CAD build for the part. Positions are in the model's coordinates, mm. A direction names the side the tool comes from. Give positions to 0.01 mm unless a question says otherwise; leave off trailing zeros. Loops run counter-clockwise (first coordinate to the right, second up) from the corner with the lowest first, then second, coordinate; pieces in that order, holes last.
Item 1: Saw through at C-C on z = -5.5. Give the number of separate pieces and of enclosed holes in the cut face, plus the area to 3 significant figures.
Item 2: Probe probe 1 along X at (y, z) = (24.5, -7); probe 2 along X at (y, z) = (35.5, -4.25); probe 3 along Y at (x, z) = (19.5, -4) (3 decimals). List the from-to ranges inside material, lowest first.
Item 3: Drop flat-ended pins along their axis: P1, Ø2, axis at y = 38, z = -2, coming from the -X side; P2, Ø2.5, axis at x = 9.35, y = 18.04, coming from the +Z side; P3, Ø1.6, axis at x = -9.35, y = 18.04, coming from the -Z side. Give the stop position or say it passes through.
Item 4: Which spindle directions (+Z, -Z, +X, -X, +Y, -Y) get a long thin tool onto all of the face, cutting with end or side? Do faces 1 (the flat face through (-25.4, 3, -5)), 2 (the cylindrical face through (-13.424, 50.221, -6.502)), 3 (the cylindrical face through (24.37, 52.895, -7.021)), 4 (the cylindrical face through (4.44, 8.16, -4.7)). Say none if no direction does.
Item 5: Mould opens along Y. For faces 5 (the cylindrical face through (24.05, 3.22, -5.2)), 6 (the cylindrical face through (18.22, 57.83, -4.7)), 7 (the flat face through (0, 67, -7)) say: released by +Y, released by -Y, zero draft, split by the parting line, or undercut.
Item 6: Saw through at B-B on y = 36. Give the cut face in (x, z) (3 decimals), plus the area to 3 significant figures.
Item 7: Saw through at A-A on y = 59.38. Give the cut face in (x, z) (3 decimals), plus the area to 3 significant figures.
from build123d import *

# Parameters (mm, degrees)
SKETCH1_R                 = 1.5875
EXTRUDE1_DEPTH            = 9.525
SKETCH2_W                 = 12.7
SKETCH2_H                 = 44.635078528
CUT_EXTRUDE1_DEPTH        = 73.561511865
FILLET1_R                 = 6.35
CHAMFER1_SIZE             = 4.445
FILLET2_R                 = 6.35
FILLET3_R                 = 6.35
SKETCH3_R                 = 2.000000064
CUT_EXTRUDE2_DEPTH        = 67.742756192
SKETCH4_R                 = 1.016
EXTRUDE2_DEPTH            = 73.561511865
LPATTERN1_COUNT           = 3
LPATTERN1_PITCH           = 6.35
LPATTERN1_COPY_1_SKETCH_R = 1.016
LPATTERN1_COPY_1_DEPTH    = 73.561511865
LPATTERN1_COPY_2_SKETCH_R = 1.016
LPATTERN1_COPY_2_DEPTH    = 73.561511865
FILLET5_R                 = 2.54


with BuildPart() as part:
    # Sketch1 → Extrude1 (new body)
    with BuildSketch(Plane.XY):
        with BuildLine():
            Line((26.18105, 50.985078528), (26.18105, 61.92))
            ThreePointArc((26.18105, 61.92), (24.693152448, 65.512102448), (21.10105, 67))
            Line((21.10105, 67), (-21.10105, 67))
            ThreePointArc((-21.10105, 67), (-24.693152448, 65.512102448), (-26.18105, 61.92))
            Line((-26.18105, 61.92), (-26.18105, 50.985078528))
            Line((-26.18105, 50.985078528), (-12.7, 50.985078528))
            Line((-12.7, 50.985078528), (-12.7, 6.35))
            Line((-12.7, 6.35), (-25.4, 6.35))
            Line((-25.4, 6.35), (-25.4, 0))
            Line((-25.4, 0), (25.4, 0))
            Line((25.4, 0), (25.4, 6.35))
            Line((25.4, 6.35), (12.7, 6.35))
            Line((12.7, 6.35), (12.7, 50.985078528))
            Line((12.7, 50.985078528), (26.18105, 50.985078528))
        make_face()
        with Locations((-18.56105, 59.38)):
            Circle(SKETCH1_R, mode=Mode.SUBTRACT)
        with Locations((18.56105, 59.38)):
            Circle(SKETCH1_R, mode=Mode.SUBTRACT)
    extrude(amount=-EXTRUDE1_DEPTH)

    # Sketch2 → Cut-Extrude1 (cut, through all)
    with BuildSketch(Plane(origin=(0, 0, -9.525), x_dir=(-1, 0, 0), z_dir=(0, 0, -1))):
        with Locations((0, 28.667539264)):
            Rectangle(SKETCH2_W, SKETCH2_H)
    extrude(amount=-CUT_EXTRUDE1_DEPTH, mode=Mode.SUBTRACT)

    # Fillet1
    fillet1_edges = [part.edges().sort_by_distance(p)[0] for p in [
        (-26.18105, 50.985078528, -4.7625),
        (26.18105, 50.985078528, -4.7625),
    ]]
    fillet(fillet1_edges, radius=FILLET1_R)

    # Chamfer1
    chamfer1_edges = [part.edges().sort_by_distance(p)[0] for p in [
        (-16.265525, 50.985078528, 0),
        (-26.18105, 59.627539264, 0),
        (16.265525, 50.985078528, 0),
        (0, 67, 0),
        (26.18105, 59.627539264, 0),
    ]]
    chamfer(chamfer1_edges, length=CHAMFER1_SIZE)

    # Fillet2
    fillet2_edges = [part.edges().sort_by_distance(p)[0] for p in [
        (6.35, 50.985078528, -4.7625),
        (-6.35, 50.985078528, -4.7625),
        (6.35, 6.35, -4.7625),
        (-6.35, 6.35, -4.7625),
    ]]
    fillet(fillet2_edges, radius=FILLET2_R - 0.0001)  # a hair under: the kernel refuses the full size

    # Fillet3
    fillet3_edges = [part.edges().sort_by_distance(p)[0] for p in [
        (-12.7, 6.35, -4.7625),
        (12.7, 6.35, -4.7625),
    ]]
    fillet(fillet3_edges, radius=FILLET3_R)

    # Sketch3 → Cut-Extrude2 (cut, through all)
    with BuildSketch(Plane(origin=(0, 6.35, 0), x_dir=(1, 0, 0), z_dir=(0, 1, 0))):
        with Locations(Location((-22.098, 4.7625, 0), (0, 0, 270))):
            Circle(SKETCH3_R)
    cut_extrude2 = extrude(amount=-CUT_EXTRUDE2_DEPTH, mode=Mode.SUBTRACT)

    # Mirror2: Cut-Extrude2 across plane
    add(cut_extrude2.mirror(Plane(origin=(0, 0, 0), x_dir=(0, 0, 1), z_dir=(1, 0, 0))), mode=Mode.SUBTRACT)

    # Sketch4 → Extrude2 (cut, through all)
    with BuildSketch(Plane.XY):
        with Locations((9.345089473, 30.742631811)):
            Circle(SKETCH4_R)
    extrude2 = extrude(amount=-EXTRUDE2_DEPTH, mode=Mode.SUBTRACT)

    # Mirror3: Extrude2 across plane
    add(extrude2.mirror(Plane(origin=(0, 0, 0), x_dir=(0, 0, 1), z_dir=(1, 0, 0))), mode=Mode.SUBTRACT)

    # LPattern1: Extrude2 ×3
    with Locations(*[(0, -i * LPATTERN1_PITCH, 0) for i in range(1, LPATTERN1_COUNT)]):
        add(extrude2, mode=Mode.SUBTRACT)

    # LPattern1 copy 1 sketch → LPattern1 copy 1 (cut, through all)
    with BuildSketch(Plane(origin=(0, -6.35, 0), x_dir=(-1, 0, 0), z_dir=(0, 0, 1))):
        with Locations((9.345089473, -30.742631811)):
            Circle(LPATTERN1_COPY_1_SKETCH_R)
    extrude(amount=-LPATTERN1_COPY_1_DEPTH, mode=Mode.SUBTRACT)

    # LPattern1 copy 2 sketch → LPattern1 copy 2 (cut, through all)
    with BuildSketch(Plane(origin=(0, -12.7, 0), x_dir=(-1, 0, 0), z_dir=(0, 0, 1))):
        with Locations((9.345089473, -30.742631811)):
            Circle(LPATTERN1_COPY_2_SKETCH_R)
    extrude(amount=-LPATTERN1_COPY_2_DEPTH, mode=Mode.SUBTRACT)

    # Fillet5
    fillet5_edges = [part.edges().sort_by_distance(p)[0] for p in [
        (-12.7, 50.985078528, -6.985),
        (12.7, 50.985078528, -6.985),
        (-12.7, 53.207578528, -2.2225),
        (12.7, 53.207578528, -2.2225),
    ]]
    fillet(fillet5_edges, radius=FILLET5_R)


solid = part.part
Results below:
1. separate pieces: 3
1. enclosed holes: 9
1. area: 1,670 mm2
2. probe 1: x = -12.7 to -10.36, -8.33 to -6.35, 6.35 to 8.33, 10.36 to 12.7
2. probe 2: x = -12.7 to -6.35, 6.35 to 12.7
2. probe 3: y = 0 to 6.35, 51.43 to 58.1, 60.66 to 66.555
3. P1: stops at x = -12.7
3. P2: stops at z = 0
3. P3: passes through
4. face 1: +Z, -Z, -X, -Y
4. face 2: +Z, -Z, -X
4. face 3: +Z, -Z, +X
4. face 4: +Z, -Z
5. face 5: zero draft
5. face 6: undercut
5. face 7: released by +Y
6. outline: (-12.7, -9.525) - (-6.35, -9.525) - (-6.35, 0) - (-12.7, 0) - close; (6.35, -9.525) - (12.7, -9.525) - (12.7, 0) - (6.35, 0) - close
6. area: 121 mm2
7. outline: (-26.181, -9.525) - (-20.149, -9.525) - (-20.149, 0) - (-21.736, 0) - (-26.181, -4.445) - close; (-16.974, -9.525) - (16.974, -9.525) - (16.974, 0) - (-16.974, 0) - close; (20.149, -9.525) - (26.181, -9.525) - (26.181, -4.445) - (21.736, 0) - (20.149, 0) - close
7. area: 419 mm2
